from build123d import *

# Parameters (mm, degrees)
SKETCH_1_W          = 20
SKETCH_1_H          = 20
SKETCH_1_W_2        = 18
SKETCH_1_H_2        = 18
EXTRUDE_1_DEPTH     = 460
SKETCH_2_R          = 1.8
CUT_EXTRUDE_1_DEPTH = 3
SKETCH_3_R          = 1.8
CUT_EXTRUDE_2_DEPTH = 3
SKETCH_5_R          = 1.8
CUT_EXTRUDE_3_DEPTH = 3
SKETCH_6_R          = 1.8
CUT_EXTRUDE_4_DEPTH = 10
SKETCH_7_R          = 1.5
CUT_EXTRUDE_5_DEPTH = 20


with BuildPart() as part:
    # 草图1 → 凸台-拉伸1 (new body)
    with BuildSketch(Plane.XY):
        Rectangle(SKETCH_1_W, SKETCH_1_H)
        Rectangle(SKETCH_1_W_2, SKETCH_1_H_2, mode=Mode.SUBTRACT)
    extrude(amount=EXTRUDE_1_DEPTH)

    # 草图2 → 切除-拉伸1 (cut)
    with BuildSketch(Plane.ZY.offset(10)):
        with Locations((10, 0)):
            Circle(SKETCH_2_R)
    extrude(amount=-CUT_EXTRUDE_1_DEPTH, mode=Mode.SUBTRACT)

    # 草图3 → 切除-拉伸2 (cut)
    with BuildSketch(Plane.ZY.offset(10)):
        with Locations((198, 0)):
            Circle(SKETCH_3_R)
    extrude(amount=-CUT_EXTRUDE_2_DEPTH, mode=Mode.SUBTRACT)

    # 草图5 → 切除-拉伸3 (cut)
    with BuildSketch(Plane.ZY.offset(10)):
        with Locations((450, 0)):
            Circle(SKETCH_5_R)
    extrude(amount=-CUT_EXTRUDE_3_DEPTH, mode=Mode.SUBTRACT)

    # 草图6 → 切除-拉伸4 (cut)
    with BuildSketch(Plane.ZY.offset(10)):
        with Locations((262, 0)):
            Circle(SKETCH_6_R)
    extrude(amount=-CUT_EXTRUDE_4_DEPTH, mode=Mode.SUBTRACT)

    # 草图7 → 切除-拉伸5 (cut)
    with BuildSketch(Plane(origin=(0, 10, 0), x_dir=(1, 0, 0), z_dir=(0, 1, 0))):
        with Locations((4, -166)):
            Circle(SKETCH_7_R)
        with Locations((-6, -166)):
            Circle(SKETCH_7_R)
        with Locations((4, -178)):
            Circle(SKETCH_7_R)
        with Locations((-6, -178)):
            Circle(SKETCH_7_R)
    extrude(amount=-CUT_EXTRUDE_5_DEPTH, mode=Mode.SUBTRACT)


solid = part.part
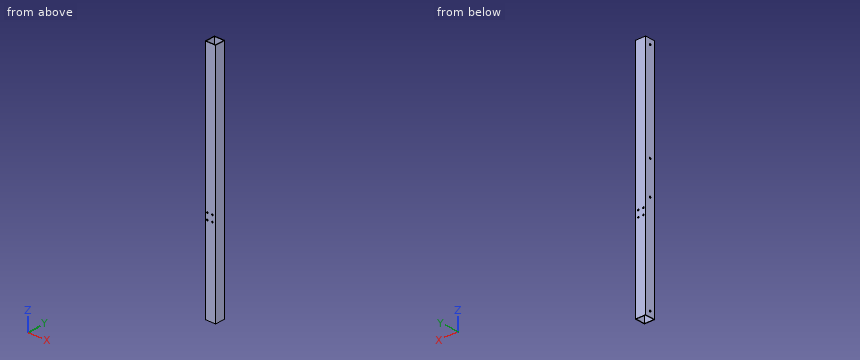
Part model, mm, in its own coordinate system. Round coordinates to 2 decimals unless told otherwise and drop trailing zeros. Order: outer loops, then holes, each group sorted by start corner. A loop starts at its lowest first (then second) coordinate and runs counter-clockwise, first axis right, second up. Notation, with made-up numbers: (19, 88.25) -> (34, 88.25) arc R19 cw to (34, 111.25) -> close; hole circle Ø8 at (53.5, -21.5). An arc over 180 degrees is marked (long way). Put each result on its own line as item: value.
Q1. Wall check: line 1 (X direction, y = 9.3, z = 178); line 2 (Z direction, x = 4, y = -9.5); line 3 (Y direction, x = -3.5, z = 335). Give the ranges that are in metal, low to high. Write a range as [from, to].
From the geometry:
line 1: x = [-10, -7.5], [-4.5, 2.5], [5.5, 10]
line 2: z = [0, 164.5], [167.5, 176.5], [179.5, 460]
line 3: y = [-10, -9], [9, 10]
Q2. Band-saw the part on A-A (z = 135.5). Give the cut face in (x, y), and give its area (3 significant figures).
From the geometry:
outline: (-10, -10) -> (10, -10) -> (10, 10) -> (-10, 10) -> close; hole (-9, -9) -> (9, -9) -> (9, 9) -> (-9, 9) -> close
area: 76.0 mm2
Q3. Pin check, flat tips, straight feed: pin 1 Ø2.5 at (x, z) = (-6, 178) entering from -Y; pin 2 Ø3 at (y, z) = (0, 198) entering from -X. Stop position of each tip, or through.
From the geometry:
pin 1: passes through
pin 2: stops at x = 9
